Check sheet for the drawn part. Datum: minimum x, y, z corner. Units: mm. A direction names the side the tool comes from. Coordinates: 2 decimals unless noted, no trailing zeros. Loops run counter-clockwise (first coordinate to the right, second up) from the corner with the lowest first, then second, coordinate; pieces in that order, holes last.
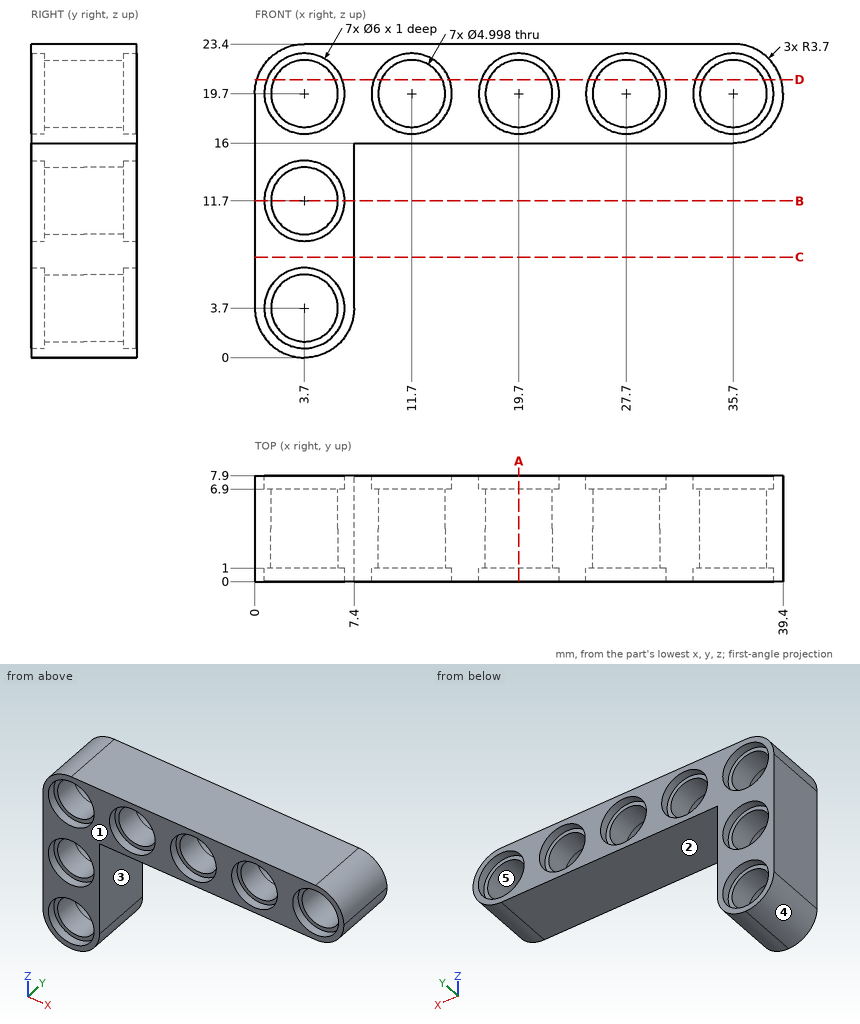
(1) Sectioned sample at B-B on z = 11.7. Record the cut outline in (x, y).
Findings:
outline: (0, 0) - (0.7, 0) - (0.7, 1) - (1.2, 1) - (1.2, 6.9) - (0.7, 6.9) - (0.7, 7.9) - (0, 7.9) - close; (6.2, 1) - (6.7, 1) - (6.7, 0) - (7.4, 0) - (7.4, 7.9) - (6.7, 7.9) - (6.7, 6.9) - (6.2, 6.9) - close
(2) Scan lines: L1, parallel to Z at x = 3.7, y = 0.7; L2, parallel to X at y = 4.75, z = 21.25; L3, parallel to Z at x = 11.7, y = 0.75. Record each from-to range of solid material in increasing order.
Findings:
L1: z = 0 to 0.7, 6.7 to 8.7, 14.7 to 16.7, 22.7 to 23.4
L2: x = 0.34 to 1.74, 5.66 to 9.74, 13.66 to 17.74, 21.66 to 25.74, 29.66 to 33.74, 37.66 to 39.06
L3: z = 16 to 16.7, 22.7 to 23.4
(3) Draft check along Z on the marked faces 3, 4 and 5. Enter one of: +Z half, -Z half, draft (parallel to the pull), parting line (faces both ways), or undercut.
Findings:
face 3: draft
face 4: -Z half
face 5: undercut
(4) Access from +Z, -Z, +X, -X, +Y, -Y to the whole of each face (thin tool, end or side, straight path). Record for the marked faces 1 and 2.
Findings:
face 1: +Z, -Z, +X, -X, -Y
face 2: -Z, +X, +Y, -Y
(5) Sectioned sample at D-D on z = 20.75. State how many separate pieces and enclosed holes the cut face has, and give its area (3 significant figures).
Findings:
separate pieces: 6
enclosed holes: 0
area: 119 mm2
(6) Gauge pin test, flat ends, axial feed: pin 1 Ø1.5 at (x, z) = (19, 14) entering from +Y; pin 2 Ø2 at (y, z) = (3, 13.5) entering from +X; pin 3 Ø5.5 at (x, z) = (3.7, 3.7) entering from -Y; pin 4 Ø5.5 at (x, z) = (3.7, 11.7) entering from +Y. Record the tip position at first contact, or that the pin passes through.
Findings:
pin 1: passes through
pin 2: stops at x = 7.4
pin 3: stops at y = 1
pin 4: stops at y = 6.9
(7) Sectioned sample at C-C on z = 7.5. Record the cut outline in (x, y), and give its area (3 significant figures).
Findings:
outline: (0, 0) - (7.4, 0) - (7.4, 7.9) - (0, 7.9) - close
area: 58.5 mm2
(8) Sectioned sample at A-A on x = 19.7. Record the cut outline in (y, z).
Findings:
outline: (0, 16) - (7.9, 16) - (7.9, 16.7) - (6.9, 16.7) - (6.9, 17.2) - (1, 17.2) - (1, 16.7) - (0, 16.7) - close; (0, 22.7) - (1, 22.7) - (1, 22.2) - (6.9, 22.2) - (6.9, 22.7) - (7.9, 22.7) - (7.9, 23.4) - (0, 23.4) - close
